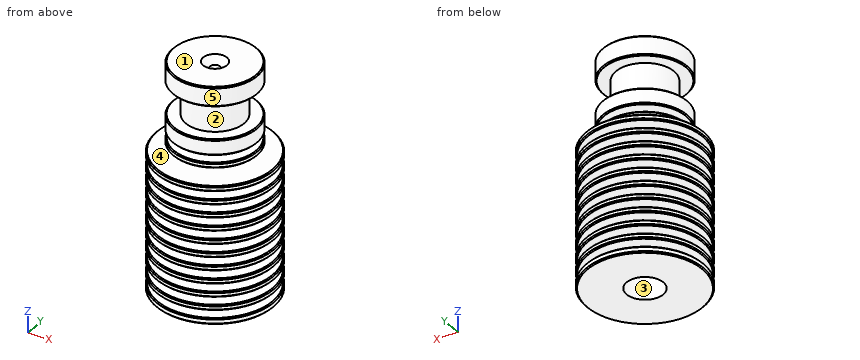
```python
from build123d import *

# Parameters (mm, degrees)
F2_SIZE = 0.2


with BuildPart() as f1:
    # F0 (on Front) → F1 (revolve)
    with BuildSketch(Plane.XZ):
        Polygon((-11.15, 0), (-3.5, 0), (-3.5, 17.3), (-1, 19.8), (-1, 41.627208), (-2.272792, 42.9), (-8, 42.9), (-8, 39.2), (-5.55, 39.2), (-5.55, 33), (-8, 33), (-8, 30), (-4.2, 30), (-4.2, 28.595), (-8, 28.595), (-8, 27.595), (-4.2, 27.595), (-4.2, 26.1), (-11.15, 26.1), (-11.15, 25.1), (-4.385, 25.1), (-4.385, 23.605), (-11.15, 23.605), (-11.15, 22.605), (-4.57, 22.605), (-4.57, 21.11), (-11.15, 21.11), (-11.15, 20.11), (-4.755, 20.11), (-4.755, 18.615), (-11.15, 18.615), (-11.15, 17.615), (-4.94, 17.615), (-4.94, 16.12), (-11.15, 16.12), (-11.15, 15.12), (-5.125, 15.12), (-5.125, 13.625), (-11.15, 13.625), (-11.15, 12.625), (-5.31, 12.625), (-5.31, 11.13), (-11.15, 11.13), (-11.15, 10.13), (-5.495, 10.13), (-5.495, 8.635), (-11.15, 8.635), (-11.15, 7.635), (-5.68, 7.635), (-5.68, 6.14), (-11.15, 6.14), (-11.15, 5.14), (-5.865, 5.14), (-5.865, 3.645), (-11.15, 3.645), (-11.15, 2.645), (-6.05, 2.645), (-6.05, 1.15), (-11.15, 1.15), align=None)
    revolve(axis=Axis((0, 0, 21.45), (0, 0, -1)))

    # F2
    f2_edges = [f1.edges().sort_by_distance(p)[0] for p in [
        (8, 0, 42.9),
        (8, 0, 39.2),
        (-8, 0, 41.05),
        (8, 0, 33),
        (8, 0, 30),
        (-8, 0, 31.5),
        (8, 0, 28.595),
        (8, 0, 27.595),
        (-8, 0, 28.095),
        (11.15, 0, 26.1),
        (11.15, 0, 25.1),
        (-11.15, 0, 25.6),
        (11.15, 0, 23.605),
        (11.15, 0, 22.605),
        (-11.15, 0, 23.105),
        (11.15, 0, 21.11),
        (11.15, 0, 20.11),
        (-11.15, 0, 20.61),
        (11.15, 0, 18.615),
        (11.15, 0, 17.615),
        (-11.15, 0, 18.115),
        (11.15, 0, 16.12),
        (11.15, 0, 15.12),
        (-11.15, 0, 15.62),
        (11.15, 0, 13.625),
        (11.15, 0, 12.625),
        (-11.15, 0, 13.125),
        (11.15, 0, 11.13),
        (11.15, 0, 10.13),
        (-11.15, 0, 10.63),
        (11.15, 0, 8.635),
        (11.15, 0, 7.635),
        (-11.15, 0, 8.135),
        (11.15, 0, 6.14),
        (11.15, 0, 5.14),
        (-11.15, 0, 5.64),
        (11.15, 0, 3.645),
        (11.15, 0, 2.645),
        (-11.15, 0, 3.145),
        (11.15, 0, 1.15),
        (11.15, 0, 0),
        (-11.15, 0, 0.575),
    ]]
    chamfer(f2_edges, length=F2_SIZE)


solid = f1.part
```
For this review, take the finished solid that the model builds, in its own axes (mm). Face numbers are marked on the shaded views. A direction names the side the tool comes from. Round coordinates to 2 decimals unless told otherwise and drop trailing zeros. Write each loop counter-clockwise with the first axis right and the second up, starting at its lowest first coordinate (ties: lowest second). Pieces come first, ordered by that corner, then holes. Notation, with made-up numbers: (-38, -25) -> (2, -25) arc R22 ccw to (2, -3) -> close; hole circle Ø7 at (35.5, -11.75). An arc over 180 degrees is marked (long way). Use one line per item in the form item = value.
Q1. Consider section B-B (x = 7.25). State how many separate pieces and enclosed holes the cut face has, then the cut area to 3 significant figures.
Resolved:
separate_pieces = 14
enclosed_holes = 0
area = 239 mm²
Q2. Clearance check with flat-ended pins moving along their axes: pin 1 Ø1 at (x, z) = (8, 35) entering from -Y; pin 2 Ø6.5 at (x, y) = (1.5, -2.5) entering from -Z; pin 3 Ø6.5 at (x, y) = (0, 0) entering from -Z; pin 4 Ø8 at (y, z) = (-7.5, 5) entering from +X. State where each tip first meets the part, or that it passes through.
Resolved:
pin_1 = through
pin_2 = 0
pin_3 = 17.55
pin_4 = 10.58
Q3. To check wall thickness, follow probe 1 along Z at (x, y) = (-0.75, -4.25) (3 decimals); probe 2 along Y at (x, z) = (0, 12); probe 3 along Y at (x, z) = (0, 6.5). State the ranges of each line that lie inside material, in increasing order. Write a range as from..to.
Resolved:
probe_1 = 0..26.1, 27.595..28.595, 30..42.9
probe_2 = -5.31..-3.5, 3.5..5.31
probe_3 = -5.68..-3.5, 3.5..5.68
Q4. Machinability: for the marked faces 1 and 2, which of the approach directions +Z, -Z, +X, -X, +Y, -Y give a long, thin tool a straight path to every point of the face, cutting with its end or side? Answer none if there is none.
Resolved:
face_1 = +Z, +X, -X, +Y, -Y
face_2 = none
Q5. The part is to be moulded in two halves that separate along Y. For the marked faces 3, 4 and 5, say which applies: released by +Y, released by -Y, zero draft, split by the parting line, or undercut.
Resolved:
face_3 = undercut
face_4 = zero draft
face_5 = split by the parting line
Q6. Consider section A-A (z = 31). State the section outline as (x, y) points.
Resolved:
outline = circle Ø16 at (0, 0); hole circle Ø2 at (0, 0)
